The model under review builds one solid part; all positions refer to its coordinate system, in mm. A direction names the side the tool comes from. Give positions to 0.01 mm unless a question says otherwise; leave off trailing zeros. Loops run counter-clockwise (first coordinate to the right, second up) from the corner with the lowest first, then second, coordinate; pieces in that order, holes last. Notation, with made-up numbers: M 68.5,19 L 118.5,19 A26 cw 118.5,51 Z; hole C 82,69.25 d5. An arc over 180 degrees is marked long. Return JSON: item names as keys, results as strings.
```python
from build123d import *

# Parameters (mm, degrees)
F1_DEPTH = 19.05
F3_DEPTH = 9.525


with BuildPart() as f1:
    # F0 (on Front) → F1 (new body)
    with BuildSketch(Plane.XZ):
        Polygon((-558.8, 0), (0, 0), (0, 825.5), (-609.6, 825.5), (-609.6, 101.6), (-558.8, 101.6), align=None)
    extrude(amount=F1_DEPTH)

    # F2 (on face) → F3 (cut)
    with BuildSketch(Plane.XZ.offset(19.05)):
        Polygon((0, 825.5), (-19.05, 825.5), (-19.05, 120.65), (-577.85, 120.65), (-577.85, 101.6), (-558.8, 101.6), (-19.05, 101.6), (-19.05, 0), (0, 0), align=None)
    extrude(amount=-F3_DEPTH, mode=Mode.SUBTRACT)


solid = f1.part
```
1) Consider section A-A on y = -14.25. Write out the cut boundary in (x, z), then the cut area to 3 significant figures.
From the geometry:
{"outline": "M -609.6,101.6 L -577.85,101.6 L -577.85,120.65 L -19.05,120.65 L -19.05,825.5 L -609.6,825.5 Z; M -558.8,0 L -19.05,0 L -19.05,101.6 L -558.8,101.6 Z", "area": "472,000 mm²"}
2) Consider section C-C on z = 668. Write out the cut boundary in (x, y) (3 decimals), then the cut area to 3 significant figures.
From the geometry:
{"outline": "M -609.6,-19.05 L -19.05,-19.05 L -19.05,-9.525 L 0,-9.525 L 0,0 L -609.6,0 Z", "area": "11,400 mm²"}
3) Wall thickness on L1, parallel to Z at x = -100, y = -10.25; L2, parallel to X at y = -16.75, z = 534; L3, parallel to X at y = -16.5, z = 120: over which ranges is each line inside the solid? List them lowest first. Write a range as from..to.
From the geometry:
{"L1": "0..101.6, 120.65..825.5", "L2": "-609.6..-19.05", "L3": "-609.6..-577.85"}
4) Consider section B-B on z = 57.5. Write out the cut boundary in (x, y) (3 decimals), then the cut area to 3 significant figures.
From the geometry:
{"outline": "M -558.8,-19.05 L -19.05,-19.05 L -19.05,-9.525 L 0,-9.525 L 0,0 L -558.8,0 Z", "area": "10,500 mm²"}
5) Tool access review of faces 1 (the face through (-590, -9, 101.6)), 2 (the face through (-609.6, -9, 469)): name each direction out of +Z, -Z, +X, -X, +Y, -Y from which nothing blocks a thin tool from reaching the whole face with its end or side.
From the geometry:
{"face 1": "-Z, -X, +Y, -Y", "face 2": "+Z, -Z, -X, +Y, -Y"}
6) Insertion check: pin 1 (3 mm diameter, centred on y = -15.5, z = 443, fed in from +X); pin 2 (5 mm diameter, centred on x = -411, z = 423.5, fed in from +Y); pin 3 (5.5 mm diameter, centred on x = -592, y = -11.5, fed in from -Z); pin 4 (3 mm diameter, centred on y = -13.5, z = 108, fed in from +X). Each pin has a flat end and moves straight along its axis. Give the tip position at first contact, or say it passes through.
From the geometry:
{"pin 1": "x = -19.05", "pin 2": "y = 0", "pin 3": "z = 101.6", "pin 4": "x = -577.85"}
